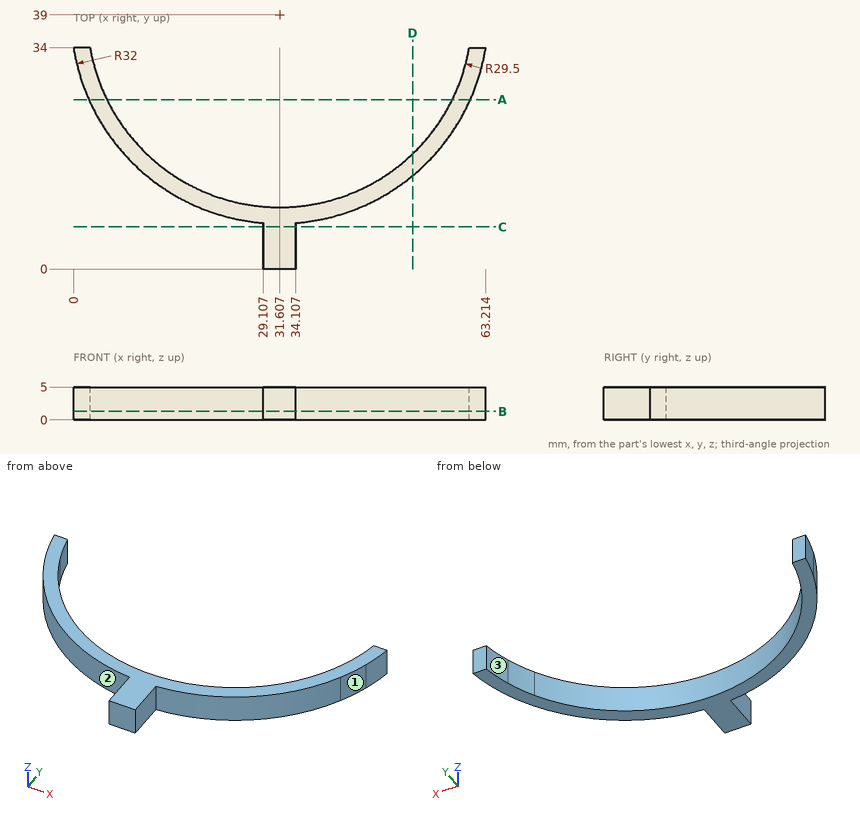
Answer from the drawing. Dimensions are ordinates in mm from the lowest x, y and z of the part. Round coordinates to 2 decimals unless told otherwise and drop trailing zeros. Write each loop counter-clockwise with the first axis right and the second up, starting at its lowest first coordinate (ties: lowest second). Pieces come first, ordered by that corner, then holes. Notation, with made-up numbers: M -13,35.25 L 2,35.25 A19 ccw 2,67.25 Z; hole C -26.75,79.5 d2. An arc over 180 degrees is marked long. Write each question's results on one line, items separated by ' | '. Start each with the question number.
Item 1: Find section D-D on x = 52. Write down the section's boundary in (y, z).
Item 2: Find section B-B on z = 1.3. Write down the section's boundary in (x, y).
Item 3: Find section C-C on y = 6.5. Write down the section's boundary in (x, z).
Item 4: Given pin 1 Ø1.5 at (y, z) = (4, 3) entering from -X; pin 2 Ø1 at (x, z) = (38.5, 2) entering from -Y (3 decimals); pin 3 Ø3 at (x, z) = (21, 1.5) entering from +Y, each flat-ended and moving along its own axis, determine where each tip first touches the part or whether it passes through.
Item 5: Straight lines are drawn through the part: probe 1 along X at (y, z) = (16.5, 2.45); probe 2 along X at (y, z) = (6.5, 4.1); probe 3 along X at (y, z) = (14.5, 0.8) (1 decimal). For each, find the intervals that lie inside material, in ascending order.
Item 6: Find section A-A on y = 26. Write down the section's boundary in (x, z), and give its area (3 significant figures).
Item 7: The mould has two halves that part along X. Classify the marked faces 1, 2 and 3: +X half, -X half, draft (parallel to the pull), parting line (faces both ways), or undercut.
Answer block:
1) outline: M 14.34,0 L 17.68,0 L 17.68,5 L 14.34,5 Z
2) outline: M 0,34 A32 ccw 1.21,29 A32 ccw 3.34,24 A32 ccw 29.11,7.1 L 29.11,0 L 34.11,0 L 34.11,7.1 A32 ccw 59.87,24 A32 ccw 62,29 A32 ccw 63.21,34 L 60.68,34 A29.5 cw 6.21,24 A29.5 cw 3.85,29 A29.5 cw 2.53,34 Z
3) outline: M 29.11,0 L 34.11,0 L 34.11,5 L 29.11,5 Z
4) pin 1: stops at x = 29.11 | pin 2: stops at y = 7.645 | pin 3: stops at y = 12.1
5) probe 1: x = 8.85 to 12.53, 50.69 to 54.36 | probe 2: x = 29.11 to 34.11 | probe 3: x = 11 to 15.2, 48 to 52.2
6) outline: M 2.37,0 L 5.13,0 L 5.13,5 L 2.37,5 Z; M 58.09,0 L 60.85,0 L 60.85,5 L 58.09,5 Z | area: 27.6 mm²
7) face 1: +X half | face 2: -X half | face 3: undercut
